Geometry check sheet. Reference: the model listing, model coordinates, mm. Face numbers are marked on the shaded views. A direction names the side the tool comes from. Coordinates: 2 decimals unless noted, no trailing zeros. Loops run counter-clockwise (first coordinate to the right, second up) from the corner with the lowest first, then second, coordinate; pieces in that order, holes last.
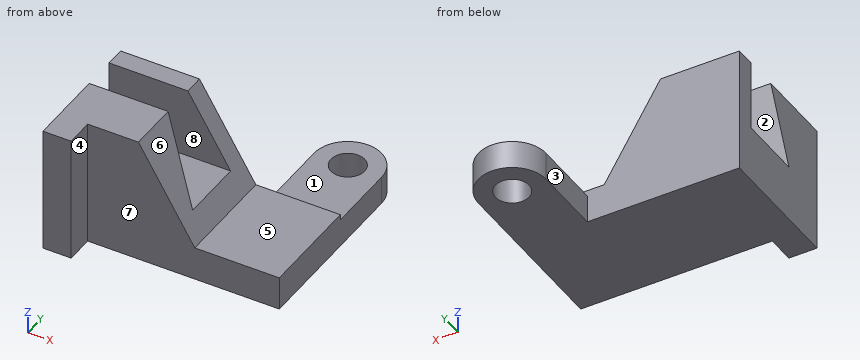
from build123d import *

# Parameters (mm, degrees)
BOSS_EXTRUDE1_DEPTH = 18.5
CUT_EXTRUDE1_DEPTH  = 92.930680406
SKETCH3_W           = 24
SKETCH3_H           = 10
BOSS_EXTRUDE2_DEPTH = 25
SKETCH4_R           = 12
SKETCH4_R_2         = 6
BOSS_EXTRUDE4_DEPTH = 10
SKETCH5_R           = 6
CUT_EXTRUDE2_DEPTH  = 102.927670433
SKETCH6_W           = 10
SKETCH6_H           = 10
BOSS_EXTRUDE5_DEPTH = 45


with BuildPart() as part:
    # Sketch1 → Boss-Extrude1 (new, symmetric)
    with BuildSketch(Plane(origin=(0, 0, 0), x_dir=(-1, 0, 0), z_dir=(0, 1, 0))):
        Polygon((0, 0), (78, 0), (78, 45), (50, 45), (30, 12), (0, 12), align=None)
    extrude(amount=BOSS_EXTRUDE1_DEPTH, both=True)

    # Sketch2 → Cut-Extrude1 (cut, through all)
    with BuildSketch(Plane(origin=(-78, 0, 0), x_dir=(0, -1, 0), z_dir=(-1, 0, 0))):
        Polygon((0.5, 45), (-11.5, 45), (-11.5, 20), (11.5, 20), align=None)
    extrude(amount=-CUT_EXTRUDE1_DEPTH, mode=Mode.SUBTRACT)

    # Sketch3 → Boss-Extrude2 (add)
    with BuildSketch(Plane(origin=(0, 18.5, 0), x_dir=(-1, 0, 0), z_dir=(0, 1, 0))):
        with Locations((12, 5)):
            Rectangle(SKETCH3_W, SKETCH3_H)
    extrude(amount=BOSS_EXTRUDE2_DEPTH)

    # Sketch4 → Boss-Extrude4 (add)
    with BuildSketch(Plane.XY.offset(10)):
        with Locations((-12, 43.5)):
            Circle(SKETCH4_R)
        with Locations((-12, 43.5)):
            Circle(SKETCH4_R_2, mode=Mode.SUBTRACT)
    extrude(amount=-BOSS_EXTRUDE4_DEPTH)

    # Sketch5 → Cut-Extrude2 (cut, through all)
    with BuildSketch(Plane.XY.offset(10)):
        with Locations((-12, 43.5)):
            Circle(SKETCH5_R)
    extrude(amount=-CUT_EXTRUDE2_DEPTH, mode=Mode.SUBTRACT)

    # Sketch6 → Boss-Extrude5 (add)
    with BuildSketch(Plane.XY.offset(45)):
        with Locations((-73, -23.5)):
            Rectangle(SKETCH6_W, SKETCH6_H)
    extrude(amount=-BOSS_EXTRUDE5_DEPTH)


solid = part.part
1) Access from +Z, -Z, +X, -X, +Y, -Y to the whole of each face (thin tool, end or side, straight path). Record for the marked faces 1, 2, 3, 4 and 5.
Data:
face 1: +Z, +X, -X, +Y
face 2: +X, -X
face 3: +Z, -Z, -X, +Y
face 4: +Z, -Z, +X, -Y
face 5: +Z, +X, +Y, -Y
2) Section check C-C on x = -64.5. Record the cut outline in (y, z), and give its area (3 significant figures).
Data:
outline: (-18.5, 0) - (18.5, 0) - (18.5, 45) - (11.5, 45) - (11.5, 20) - (-11.5, 20) - (-0.5, 45) - (-18.5, 45) - close
area: 1,230 mm2
3) Section check D-D on y = 46. Record the cut outline in (x, z).
Data:
outline: (-23.74, 0) - (-17.45, 0) - (-17.45, 10) - (-23.74, 10) - close; (-6.55, 0) - (-0.26, 0) - (-0.26, 10) - (-6.55, 10) - close
4) Section check B-B on x = -12. Record the cut outline in (y, z), and give its area (3 significant figures).
Data:
outline: (-18.5, 0) - (37.5, 0) - (37.5, 10) - (18.5, 10) - (18.5, 12) - (-18.5, 12) - close; (49.5, 0) - (55.5, 0) - (55.5, 10) - (49.5, 10) - close
area: 694 mm2
5) Material ranges on probe 1 along X at (y, z) = (43.5, 4.25); probe 2 along Y at (x, z) = (-12, 6); probe 3 along Z at (x, y) = (-26, -10), recorded low to high.
Data:
probe 1: x = -24 to -18, -6 to 0
probe 2: y = -18.5 to 37.5, 49.5 to 55.5
probe 3: z = 0 to 12
6) Depth check by flat-ended pin: pin 1 (9 mm diameter, centred on x = -21, y = -9, fed in from +Z); pin 2 (13.5 mm diameter, centred on x = -48.5, z = 12, fed in from -Y); pin 3 (1 mm diameter, centred on y = -8.5, z = 35.5, fed in from +X). Enter the tip coordinate at first touch or a pass-through.
Data:
pin 1: stops at z = 12
pin 2: stops at y = -18.5
pin 3: stops at x = -43.94
7) Mould release check, pull along Y, two halves, no side actions. Record for the marked faces 6, 7 and 8: +Y half, -Y half, draft (parallel to the pull), parting line (faces both ways), or undercut.
Data:
face 6: draft
face 7: -Y half
face 8: undercut
8) Section check A-A on z = 5. Record the cut outline in (x, y).
Data:
outline: (-78, -28.5) - (-68, -28.5) - (-68, -18.5) - (0, -18.5) - (0, 43.5) arc R12 ccw to (-24, 43.5) - (-24, 18.5) - (-78, 18.5) - close; hole circle Ø12 at (-12, 43.5)
